Autodesk Inventor part; units mm, degrees
ref_plane "YZ Plane" through (0, 0, 0) normal (1, 0, 0) x (0, 1, 0)
ref_plane "XZ Plane" through (0, 0, 0) normal (0, 1, 0) x (-1, 0, 0)
ref_plane "XY Plane" through (0, 0, 0) normal (0, 0, 1) x (1, 0, 0)
sketch "Sketch1" plane through (0, 0, 0) normal (0, 0, 1) x (1, 0, 0)
  line L0 (82, 0) -> (82, 45)
  line L1 (0, 45) -> (0, 0)
  line L2 (10, 45) -> (10, 55)
  line L3 (10, 55) -> (0, 55)
  line L4 (0, 55) -> (0, 45)
  line L5 (72, 45) -> (72, 55)
  line L6 (72, 55) -> (82, 55)
  line L7 (82, 55) -> (82, 45)
  line L8 (10, 45) -> (72, 45)
  line L9 (0, 0) -> (37.791, 0)
  line L10 (37.791, 0) -> (37.791, -10)
  line L11 (37.791, -10) -> (47.791, -10)
  line L12 (47.791, -10) -> (47.791, 0)
  line L13 (47.791, 0) -> (82, 0)
  circle A0 centre (42.843, -5.687) radius 1.6
  line L14 (0, 45) -> (0, 51)
  line L15 (82, 45) -> (82, 51)
  circle A1 centre (4.971, 51) radius 1.6
  circle A2 centre (77.029, 51) radius 1.6
  dimension "d0" = 82
  dimension "d1" = 45
  dimension "d2" = 10
  dimension "d3" = 10
  dimension "d4" = 10
  dimension "d5" = 10
  dimension "d10" = 37.791
  dimension "d11" = 10
  dimension "d12" = 10
  dimension "d15" = 3.2
  dimension "d16" = 6
  dimension "d20" = 3.2
  dimension "d21" = 3.2
extrude "Extrusion1" add sketch "Sketch1" along normal blind 4
sketch "Sketch3" plane through (0, 0, 4) normal (0, 0, 1) x (1, 0, 0)
  circle A0 centre (4.971, 51) radius 1.6
  circle A1 centre (4.971, 51) radius 2.75
  circle A2 centre (77.029, 51) radius 1.6
  circle A3 centre (77.029, 51) radius 2.75
  circle A4 centre (42.843, -5.687) radius 1.6
  circle A5 centre (42.843, -5.687) radius 2.75
  point P0 (0, 0)
  dimension "d24" = 5.5
  dimension "d25" = 5.5
  dimension "d26" = 5.5
extrude "Extrusion2" cut sketch "Sketch3" against normal blind 2.5
sketch "Sketch4" plane through (0, 0, 4) normal (0, 0, 1) x (1, 0, 0)
  line L0 (10, 55) -> (0, 55)
  line L1 (10, 45) -> (10, 55)
  line L2 (0, 55) -> (10, 55)
  line L3 (10, 55) -> (10, 54.5)
  line L4 (10, 54.5) -> (0, 54.5)
  line L5 (0, 54.5) -> (0, 55)
  line L6 (0, 0) -> (0, 55)
  line L7 (0, 0) -> (37.791, 0)
  line L8 (0, 55) -> (0.5, 55)
  line L9 (0.5, 55) -> (0.5, 0)
  line L10 (0.5, 0) -> (0, 0)
  line L11 (0, 0) -> (0, 55)
  line L12 (0, 0) -> (37.791, 0)
  line L13 (37.791, 0) -> (37.791, 0.5)
  line L14 (37.791, 0.5) -> (0, 0.5)
  line L15 (0, 0.5) -> (0, 0)
  line L16 (37.791, 0) -> (37.791, -10)
  line L17 (37.791, -10) -> (38.291, -10)
  line L18 (38.291, -10) -> (38.291, 0.5)
  line L19 (38.291, 0.5) -> (37.791, 0.5)
  line L20 (37.791, 0.5) -> (37.791, -10)
  line L21 (47.791, 0) -> (47.791, -10)
  line L22 (37.791, -10) -> (47.791, -10)
  line L23 (47.791, -10) -> (47.791, -9.5)
  line L24 (47.791, -9.5) -> (37.791, -9.5)
  line L25 (37.791, -9.5) -> (37.791, -10)
  line L26 (47.791, -10) -> (47.291, -10)
  line L27 (47.291, -10) -> (47.291, 0.5)
  line L28 (47.291, 0.5) -> (47.791, 0.5)
  line L29 (47.791, 0.5) -> (47.791, -10)
  line L30 (82, 0) -> (82, 55)
  line L31 (47.291, 0.5) -> (82, 0.5)
  line L32 (82, 0.5) -> (82, 0)
  line L33 (82, 0) -> (47.291, 0)
  line L34 (47.291, 0) -> (47.291, 0.5)
  line L35 (82, 55) -> (72, 55)
  line L36 (82, 0) -> (81.5, 0)
  line L37 (81.5, 0) -> (81.5, 55)
  line L38 (81.5, 55) -> (82, 55)
  line L39 (82, 55) -> (82, 0)
  line L40 (72, 55) -> (72, 45)
  line L41 (82, 55) -> (72, 55)
  line L42 (72, 55) -> (72, 54.5)
  line L43 (72, 54.5) -> (82, 54.5)
  line L44 (82, 54.5) -> (82, 55)
  line L45 (10, 45) -> (72, 45)
  line L46 (10, 45) -> (72, 45)
  line L47 (72, 45) -> (72, 44.5)
  line L48 (72, 44.5) -> (10, 44.5)
  line L49 (10, 44.5) -> (10, 45)
  line L50 (72, 44.5) -> (72.5, 44.5)
  line L51 (72.5, 44.5) -> (72.5, 55)
  line L52 (72.5, 55) -> (72, 55)
  line L53 (72, 55) -> (72, 44.5)
  line L54 (10, 44.5) -> (9.5, 44.5)
  line L55 (9.5, 44.5) -> (9.5, 55)
  line L56 (9.5, 55) -> (10, 55)
  line L57 (10, 55) -> (10, 44.5)
  dimension "d30" = 0.5
  dimension "d31" = 0.5
  dimension "d32" = 0.5
  dimension "d33" = 0.5
  dimension "d34" = 0.5
  dimension "d35" = 0.5
  dimension "d36" = 0.5
  dimension "d37" = 0.5
  dimension "d38" = 0.5
  dimension "d39" = 0.5
  dimension "d40" = 0.5
extrude "Extrusion3" cut sketch "Sketch4" against normal blind 10 contours L1 L4 L55 L0 | L55 L4 L9 L0 | L1 L49 L54 L55 L4 | L9 L4 L5 L0 | L45 L47 L48 L49 | L9 L14 L6 L4 | L40 L43 L51 L50 L47 | L14 L13 L7 L9 | L9 L7 L6 L14 | L40 L35 L51 L43 | L19 L18 L24 L16 L13 | L51 L35 L37 L43 | L43 L30 L31 L37 | L37 L35 L30 L43 | L24 L18 L17 L16 | L24 L27 L22 L18 | L37 L33 L29 L31 | L31 L30 L33 L37 | L27 L33 L21 L24 | L24 L21 L22 L27 | L29 L33 L27 L28
fillet "Fillet2" radius 2 2 edges at (0.5, 27.5, 4) (81.5, 27.5, 4)
properties part number "battery_cover"
Input: part model. Units: mm. Frame: model coordinates. A direction names the side the tool comes from. Coordinates: 2 decimals unless noted, no trailing zeros. Write each loop counter-clockwise with the first axis right and the second up, starting at its lowest first coordinate (ties: lowest second). Pieces come first, ordered by that corner, then holes.
1) Material intervals for line 1 along X through (y, z) = (46, 0.45); line 2 along X through (y, z) = (52, 3.4); line 3 along X through (y, z) = (-2, 3.5), sorted ascending.
2) Section A-A on y = -2. Output: boundary loops of the cut face in (x, z), and give its area (3 significant figures).
3) Pin query (flat end, axial travel): pin 1 Ø4 at (x, y) = (77.029, 51) entering from +Z; pin 2 Ø2 at (y, z) = (-2.5, 2.5) entering from +X; pin 3 Ø1.2 at (x, z) = (53.5, 2) entering from +Y. Return the tip coordinate at first contact, or that it passes through.
4) Section B-B on x = 68.5. Output: boundary loops of the cut face in (y, z).
5) Mould query, pull axis X, two halves, no side actions, for faces 6 (the cylindrical face through (78.555, 50.519, 0.74)), 7 (the cylindrical face through (1.1, 24.8, 3.43)), 8 (the flat face through (9.5, 49, 2)), 9 (the flat face through (40, 23, 0)). Classes: pulls with the +X half, pulls with the -X half, needs draft (parallel to the pull), parting line crosses it, or undercut.
6) Set-up query: faces 1 (the flat face through (7, 51, 1.5)), 2 (the flat face through (47.291, -5, 2)), 3 (the flat face through (72.5, 49, 2)), 4 (the flat face through (38.291, -5, 2)), 5 (the flat face through (43, -9.5, 2)). Return all of +Z, -Z, +X, -X, +Y, -Y with unobstructed straight access to the full face (end or side cutting, diameter ignored); none if empty.
Check result:
1. line 1: x = 0.5 to 9.5, 72.5 to 81.5
1. line 2: x = 1.07 to 2.41, 7.53 to 9.5, 72.5 to 74.47, 79.59 to 80.93
1. line 3: x = 38.29 to 47.29
2. outline: (38.29, 0) - (47.29, 0) - (47.29, 4) - (38.29, 4) - close
2. area: 36.0 mm2
3. pin 1: stops at z = 1.5
3. pin 2: stops at x = 47.29
3. pin 3: stops at y = 44.5
4. outline: (0.5, 0) - (44.5, 0) - (44.5, 4) - (0.5, 4) - close
5. face 6: undercut
5. face 7: pulls with the -X half
5. face 8: undercut
5. face 9: needs draft
6. face 1: +Z
6. face 2: +Z, -Z, +X, -Y
6. face 3: +Z, -Z, +Y
6. face 4: +Z, -Z, -X, -Y
6. face 5: +Z, -Z, +X, -X, -Y
